Could you check a few things on this drawing? It's one solid part, dimensions in mm from its lowest x, y, z. Round coordinates to 2 decimals unless told otherwise and drop trailing zeros. Loops run counter-clockwise (first coordinate to the right, second up) from the corner with the lowest first, then second, coordinate; pieces in that order, holes last. Notation, with made-up numbers: (-11, -26) -> (6, -26) arc R31 cw to (6, 8) -> close; hole circle Ø2 at (88.5, 78.25). An arc over 180 degrees is marked (long way). Write each question's results on one line, items separated by ' | '.
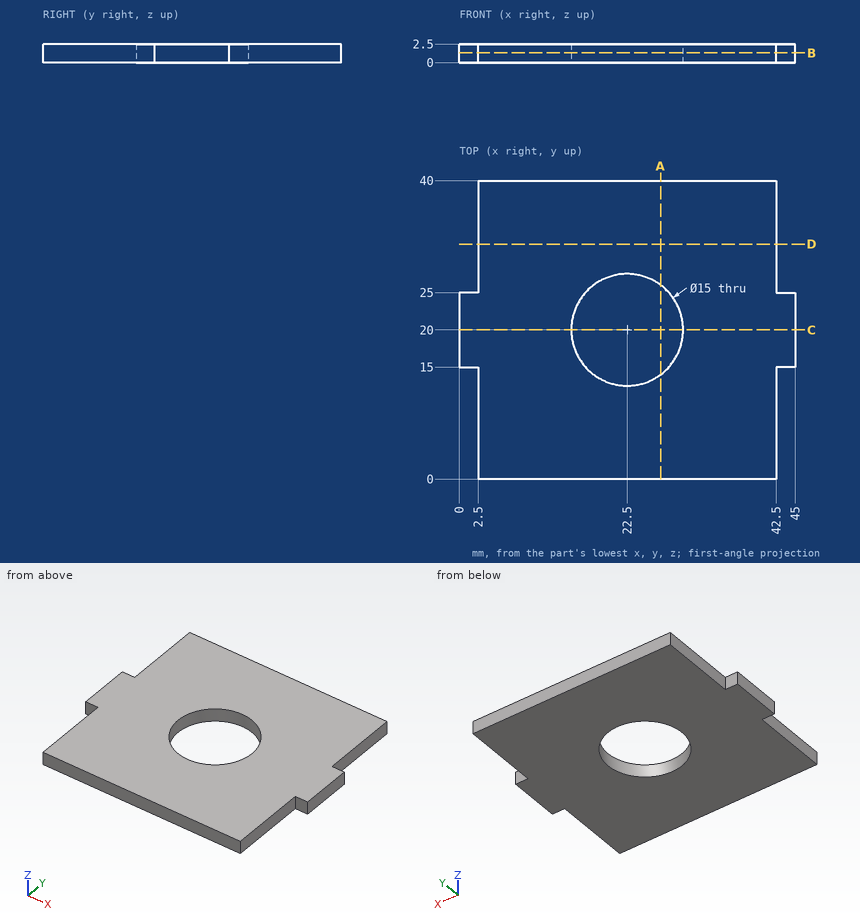
1) I want a section at B-B, the plane z = 1.3. Write out the boundary of the cut face in (x, y).
Model answer:
outline: (0, 15) -> (2.5, 15) -> (2.5, 0) -> (42.5, 0) -> (42.5, 15) -> (45, 15) -> (45, 25) -> (42.5, 25) -> (42.5, 40) -> (2.5, 40) -> (2.5, 25) -> (0, 25) -> close; hole circle Ø15 at (22.5, 20)
2) I want a section at D-D, the plane y = 31.5. Write out the boundary of the cut face in (x, z), plus the area to 3 significant figures.
Model answer:
outline: (2.5, 0) -> (42.5, 0) -> (42.5, 2.5) -> (2.5, 2.5) -> close | area: 100 mm2
3) I want a section at C-C, the plane y = 20. Write out the boundary of the cut face in (x, z).
Model answer:
outline: (0, 0) -> (15, 0) -> (15, 2.5) -> (0, 2.5) -> close; (30, 0) -> (45, 0) -> (45, 2.5) -> (30, 2.5) -> close
4) I'm going to push flat-ended pins straight in: pin 1 (0.8 mm diameter, centred on x = 1, z = 1.5, fed in from -Y); pin 2 (13.5 mm diameter, centred on x = 22.5, y = 20, fed in from -Z); pin 3 (0.8 mm diameter, centred on y = 35, z = 1, fed in from +X). Where does each tip first touch, or does it pass through?
Model answer:
pin 1: stops at y = 15 | pin 2: passes through | pin 3: stops at x = 42.5
5) I need wall thicknesses on line 1 (Y direction, x = 22.5, z = 0.6); line 2 (X direction, y = 11, z = 1.5); line 3 (X direction, y = 18, z = 0.7). Which ranges of each line are inside material? Lowest first, please.
Model answer:
line 1: y = 0 to 12.5, 27.5 to 40 | line 2: x = 2.5 to 42.5 | line 3: x = 0 to 15.27, 29.73 to 45
6) I want a section at A-A, the plane x = 27. Write out the boundary of the cut face in (y, z).
Model answer:
outline: (0, 0) -> (14, 0) -> (14, 2.5) -> (0, 2.5) -> close; (26, 0) -> (40, 0) -> (40, 2.5) -> (26, 2.5) -> close
